Geometry check sheet. Reference: the model listing, model coordinates, mm. A direction names the side the tool comes from. Coordinates: 2 decimals unless noted, no trailing zeros. Loops run counter-clockwise (first coordinate to the right, second up) from the corner with the lowest first, then second, coordinate; pieces in that order, holes last. Notation, with made-up numbers: M -36,63 L 10,63 A24 cw 10,86 Z; hole C -30,85 d11. An arc over 180 degrees is marked long. One line per question, with ' | ' between items. Start each with the question number.
from build123d import *

# Parameters (mm, degrees)
SKETCH1_R          = 5.0038
BASE_EXTRUDE_DEPTH = 21.971
CUT_EXTRUDE1_DEPTH = 15.113


with BuildPart() as part:
    # Sketch1 → Base-Extrude (new body)
    with BuildSketch(Plane.XY):
        with BuildLine():
            ThreePointArc((2.465672848, 12.801965086), (0, 14.732), (-2.465672848, 12.801965086))
            ThreePointArc((-2.465672848, 12.801965086), (-6.195465294, 6.195465294), (-12.801965086, 2.465672848))
            ThreePointArc((-12.801965086, 2.465672848), (-14.732, 0), (-12.801965086, -2.465672848))
            ThreePointArc((-12.801965086, -2.465672848), (-6.195465294, -6.195465294), (-2.465672848, -12.801965086))
            ThreePointArc((-2.465672848, -12.801965086), (0, -14.732), (2.465672848, -12.801965086))
            ThreePointArc((2.465672848, -12.801965086), (6.195465294, -6.195465294), (12.801965086, -2.465672848))
            ThreePointArc((12.801965086, -2.465672848), (14.732, 0), (12.801965086, 2.465672848))
            ThreePointArc((12.801965086, 2.465672848), (6.195465294, 6.195465294), (2.465672848, 12.801965086))
        make_face()
        Circle(SKETCH1_R, mode=Mode.SUBTRACT)
    extrude(amount=BASE_EXTRUDE_DEPTH)

    # Sketch2 → Cut-Extrude1 (cut)
    with BuildSketch(Plane.XY.offset(21.971)):
        with BuildLine():
            Line((-8.197404848, 2.032), (8.197404848, 2.032))
            ThreePointArc((8.197404848, 2.032), (8.4455, 0), (8.197404848, -2.032))
            Line((8.197404848, -2.032), (-8.197404848, -2.032))
            ThreePointArc((-8.197404848, -2.032), (-8.4455, 0), (-8.197404848, 2.032))
        make_face()
    extrude(amount=-CUT_EXTRUDE1_DEPTH, mode=Mode.SUBTRACT)


solid = part.part
1. Sectioned sample at D-D (y = -3). Record the cut outline in (x, z), and give its area (3 significant figures).
2. Sectioned sample at B-B (x = 0). Record the cut outline in (y, z), and give its area (3 significant figures).
3. Draft check along X on faces 1 (the cylindrical face through (6.12, -6.27, 10.83)), 2 (the flat face through (6, 2.032, 15)), 3 (the flat face through (-1.2, -5.4, 21.971)). Enter one of: +X half, -X half, draft (parallel to the pull), parting line (faces both ways), or undercut.
4. Tool access check on faces 4 (the cylindrical face through (-6.27, -6.12, 10.83)), 5 (the flat face through (7, 0, 6.858)). Record the directions out of +Z, -Z, +X, -X, +Y, -Y that give a thin tool (end or side, any length) a straight path to the whole face; none if there is none.
5. Sectioned sample at C-C (z = 11.75). Record the cut outline in (x, y), and give its area (3 significant figures).
6. Sectioned sample at A-A (y = 0). Record the cut outline in (x, z), and give its area (3 significant figures).
7. Thickness scan on line 1 (X direction, y = 0, z = 7.75); line 2 (Y direction, x = 0, z = 16.5); line 3 (Y direction, x = 1.25, z = 6.5). Record the ranges inside material, lowest first.
8. Depth check by flat-ended pin: pin 1 Ø1.8 at (x, z) = (-6, 15.5) entering from +Y; pin 2 Ø1.8 at (x, z) = (6.5, 13) entering from -Y; pin 3 Ø3 at (y, z) = (-2, 8.5) entering from +X. Enter the tip coordinate at first touch or a pass-through.
Result:
1) outline: M -11.11,0 L -4,0 L -4,21.97 L -11.11,21.97 Z; M 4,0 L 11.11,0 L 11.11,21.97 L 4,21.97 Z | area: 312 mm2
2) outline: M -14.73,0 L -5,0 L -5,21.97 L -14.73,21.97 Z; M 5,0 L 14.73,0 L 14.73,21.97 L 5,21.97 Z | area: 427 mm2
3) face 1: +X half | face 2: undercut | face 3: draft
4) face 4: +Z, -Z, -X, -Y | face 5: +Z
5) outline: M -12.8,-2.47 A14.15 cw -2.47,-12.8 A2.54 ccw 2.47,-12.8 A14.15 cw 12.8,-2.47 A2.54 ccw 12.8,2.47 A14.15 cw 2.47,12.8 A2.54 ccw -2.47,12.8 A14.15 cw -12.8,2.47 A2.54 ccw Z; hole M -8.2,-2.03 L -4.57,-2.03 A5 ccw 4.57,-2.03 L 8.2,-2.03 A8.45 ccw 8.2,2.03 L 4.57,2.03 A5 ccw -4.57,2.03 L -8.2,2.03 A8.45 ccw Z | area: 283 mm2
6) outline: M -14.73,0 L -5,0 L -5,6.86 L -8.45,6.86 L -8.45,21.97 L -14.73,21.97 Z; M 5,0 L 14.73,0 L 14.73,21.97 L 8.45,21.97 L 8.45,6.86 L 5,6.86 Z | area: 323 mm2
7) line 1: x = -14.73 to -8.45, 8.45 to 14.73 | line 2: y = -14.73 to -5, 5 to 14.73 | line 3: y = -14.4 to -4.85, 4.85 to 14.4
8) pin 1: stops at y = 7.43 | pin 2: stops at y = -6.83 | pin 3: stops at x = 14.68
